```python
from build123d import *

# Parameters (mm, degrees)
F0_W     = 7.4329227209
F0_H     = 2.4776421487
F0_W_2   = 7.4329264462
F1_DEPTH = 8
F3_DEPTH = 30
F5_DEPTH = 30


with BuildPart() as f1:
    # F0 (on Front) → F1 (new body)
    with BuildSketch(Plane.XZ):
        with Locations((-25.923974812, -41.8709013611)):
            Rectangle(F0_W, F0_H)
        Polygon((-19.7298713028, -43.1097224355), (-19.7298713028, 62.3026564717), (-22.2075134516, 62.3026564717), (-22.2075134516, -40.6320802867), (-22.2075134516, -43.1097224355), align=None)
        Polygon((-19.7298713028, 64.7802948952), (-71.3098570704, 64.7802948952), (-71.3098570704, 62.3026564717), (-68.832218647, 62.3026564717), (-22.2075134516, 62.3026564717), (-19.7298713028, 62.3026564717), align=None)
        Polygon((-68.832218647, 62.3026564717), (-71.3098570704, 62.3026564717), (-71.3098570704, -43.1097224355), (-68.832218647, -43.1097224355), (-68.832218647, -40.6320802867), align=None)
        with Locations((-65.1157554239, -41.8709013611)):
            Rectangle(F0_W_2, F0_H)
    extrude(amount=F1_DEPTH)

    # F2 (on face) → F3 (join)
    with BuildSketch(Plane(origin=(0, 0, 0), x_dir=(-1, 0, 0), z_dir=(0, 1, 0))):
        Polygon((71.3098570704, 64.7802948952), (19.7298713028, 64.7802948952), (19.7298713028, 62.3026564717), (22.2075134516, 62.3026564717), (68.832218647, 62.3026564717), (71.3098570704, 62.3026564717), align=None)
    extrude(amount=F3_DEPTH)

    # F4 (on face) → F5 (join)
    with BuildSketch(Plane.XZ.offset(8)):
        Polygon((-19.7298713028, 64.7802948952), (-71.3098570704, 64.7802948952), (-71.3098570704, 62.3026564717), (-68.832218647, 62.3026564717), (-22.2075134516, 62.3026564717), (-19.7298713028, 62.3026564717), align=None)
    extrude(amount=F5_DEPTH)


solid = f1.part
```
CAD build for the part. Positions are in the model's coordinates, mm. A direction names the side the tool comes from. Coordinates: 2 decimals unless noted, no trailing zeros. Order: outer loops, then holes, each group sorted by start corner. A loop starts at its lowest first (then second) coordinate and runs counter-clockwise, first axis right, second up. Notation, with made-up numbers: (8.5, -22.5) -> (22.5, -22.5) arc R15 cw to (22.5, 1.5) -> close; hole circle Ø2 at (-14.75, 37.5). An arc over 180 degrees is marked (long way). Use one line per item in the form item = value. Start each with the question number.
1) Band-saw the part on D-D on x = -34. Give the cut face in (y, z), then the cut area to 3 significant figures.
2) Drop flat-ended pins along their axis: pin 1 (15.5 mm diameter, centred on x = -38, y = -14.5, fed in from -Z); pin 2 (10 mm diameter, centred on y = -14, z = 6.5, fed in from -X); pin 3 (8 mm diameter, centred on x = -65.5, z = 35, fed in from +Y); pin 4 (8 mm diameter, centred on x = -23.5, z = -16, fed in from -Y). Give the stop position or say it passes through.
3) Pull direction X, two halves, no side cores. Call faces 1 (the flat face through (-19.73, -4, 23)), 2 (the flat face through (-26, -4, -40.632)), 3 (the flat face through (-71.31, -1, 23)), 4 (the flat face through (-21, -8, 6)): +X half, -X half, draft (parallel to the pull), parting line (faces both ways), or undercut.
4) Band-saw the part on A-A on z = -2. Give the cut face in (x, y).
5) Tool access for faces 5 (the flat face through (-69, 0, 6)), 6 (the flat face through (-22.208, -4, 12)), 7 (the flat face through (-69, -8, 6)), 8 (the flat face through (-61.399, -4, -42)): list every direction of +Z, -Z, +X, -X, +Y, -Y with a clear straight run to the whole face (end or side of a thin tool).
6) Band-saw the part on C-C on y = -1.5. Give the cut face in (x, z).
7) Drill centre lines: L1, parallel to Z at x = -29, y = -2; L2, parallel to X at y = -5, z = 44; L3, parallel to Z at x = -48, y = -2. Where is each one in solid material? Low to high. Write a range as [from, to].
8) Band-saw the part on B-B on x = -62.5. Give the cut face in (y, z), then the cut area to 3 significant figures.
Entries:
q1.outline = (-38, 62.3) -> (30, 62.3) -> (30, 64.78) -> (-38, 64.78) -> close
q1.area = 168 mm2
q2.pin_1 = 62.3
q2.pin_2 = through
q2.pin_3 = 0
q2.pin_4 = -8
q3.face_1 = +X half
q3.face_2 = undercut
q3.face_3 = -X half
q3.face_4 = draft
q4.outline = (-71.31, -8) -> (-68.83, -8) -> (-68.83, 0) -> (-71.31, 0) -> close; (-22.21, -8) -> (-19.73, -8) -> (-19.73, 0) -> (-22.21, 0) -> close
q5.face_5 = -Z, +X, -X, +Y
q5.face_6 = +Y, -Y
q5.face_7 = -Z, +X, -X, -Y
q5.face_8 = -Z, +Y, -Y
q6.outline = (-71.31, -43.11) -> (-61.4, -43.11) -> (-61.4, -40.63) -> (-68.83, -40.63) -> (-68.83, 62.3) -> (-22.21, 62.3) -> (-22.21, -40.63) -> (-29.64, -40.63) -> (-29.64, -43.11) -> (-19.73, -43.11) -> (-19.73, 64.78) -> (-71.31, 64.78) -> close
q7.L1 = [-43.11, -40.63], [62.3, 64.78]
q7.L2 = [-71.31, -68.83], [-22.21, -19.73]
q7.L3 = [62.3, 64.78]
q8.outline = (-38, 62.3) -> (30, 62.3) -> (30, 64.78) -> (-38, 64.78) -> close; (-8, -43.11) -> (0, -43.11) -> (0, -40.63) -> (-8, -40.63) -> close
q8.area = 188 mm2
